```python
from build123d import *

# Parameters (mm, degrees)
SKETCH1_R               = 10
SKETCH1_R_2             = 4
BOSS_EXTRUDE1_DEPTH     = 30
SKETCH2_R               = 2
CUT_EXTRUDE1_DEPTH      = 11
CUT_EXTRUDE1_DEPTH_BACK = 11
FILLET1_R               = 1


with BuildPart() as part:
    # Sketch1 → Boss-Extrude1 (new body)
    with BuildSketch(Plane(origin=(0, 0, 0), x_dir=(1, 0, 0), z_dir=(0, 1, 0))):
        Circle(SKETCH1_R)
        Circle(SKETCH1_R_2, mode=Mode.SUBTRACT)
    extrude(amount=BOSS_EXTRUDE1_DEPTH)

    # Sketch2 → Cut-Extrude1 (cut, two sides)
    with BuildSketch(Plane(origin=(0, 0, 0), x_dir=(0, 0, -1), z_dir=(1, 0, 0))) as cut_extrude1_sk:
        with Locations((6.5, 25.5)):
            Circle(SKETCH2_R)
        with Locations((-6.5, 4.5)):
            Circle(SKETCH2_R)
    extrude(amount=CUT_EXTRUDE1_DEPTH, mode=Mode.SUBTRACT)
    extrude(cut_extrude1_sk.sketch, amount=-CUT_EXTRUDE1_DEPTH_BACK, mode=Mode.SUBTRACT)

    # Fillet1
    fillet1_edges = [part.edges().sort_by_distance(p)[0] for p in [
        (-10, 0, 0),
        (-10, 30, 0),
        (-4, 0, 0),
        (-4, 30, 0),
    ]]
    fillet(fillet1_edges, radius=FILLET1_R)


solid = part.part
```
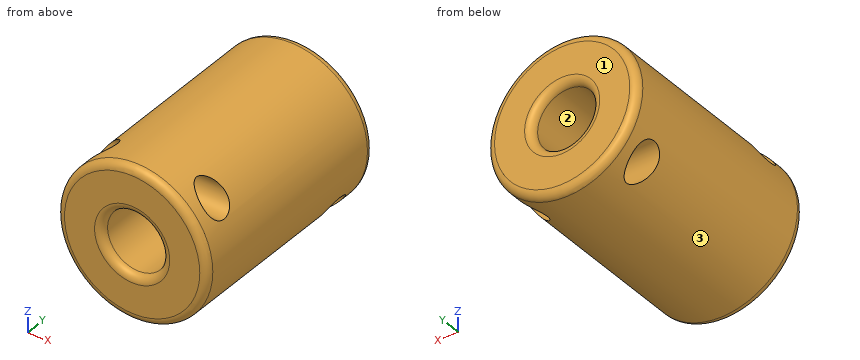
Source: CAD feature listing. Evaluate the final solid. Frame: model axes, mm. Face numbers are marked on the shaded views. Give positions to 0.01 mm unless a question says otherwise; leave off trailing zeros. Write each loop counter-clockwise with the first axis right and the second up, starting at its lowest first coordinate (ties: lowest second). Pieces come first, ordered by that corner, then holes.
1. Section query A-A (z = 0). Return the cut outline in (x, y).
2. Section query C-C (x = -2.25). Count the separate pieces of the cut face and the enclosed holes in it, then the cut area to 3 significant figures.
3. First-contact query: pin 1 (12 mm diameter, centred on x = -7, y = 6.5, fed in from +Z); pin 2 (1.5 mm diameter, centred on x = 4, y = 17, fed in from +Z); pin 3 (5 mm diameter, centred on y = 4.5, z = 6.5, fed in from -X); pin 4 (3.5 mm diameter, centred on y = 25.5, z = -6.5, fed in from -X). Flat tips, straight axial feed; report the tip coordinate or a pass-through.
4. Section query D-D (y = 21). Return the cut outline in (x, z).
5. Pull-direction query (Z, two-part tool) for the marked faces 1, 2 and 3; classes: +Z half, -Z half, draft (parallel to the pull), parting line (faces both ways), or undercut.
6. Material intervals for line 1 along Y through (x, z) = (6.25, 6.5); line 2 along Y through (x, z) = (-3.25, -6.5); line 3 along X through (y, z) = (3, 0), sorted ascending.
7. Section query B-B (y = 3.25). Return the cut outline in (x, z).
Output values:
1. outline: (-10, 1) arc R1 ccw to (-9, 0) - (-5, 0) arc R1 ccw to (-4, 1) - (-4, 29) arc R1 ccw to (-5, 30) - (-9, 30) arc R1 ccw to (-10, 29) - close; (4, 1) arc R1 ccw to (5, 0) - (9, 0) arc R1 ccw to (10, 1) - (10, 29) arc R1 ccw to (9, 30) - (5, 30) arc R1 ccw to (4, 29) - close
2. separate pieces: 2
2. enclosed holes: 2
2. area: 359 mm2
3. pin 1: stops at z = 9.95
3. pin 2: stops at z = 9.46
3. pin 3: stops at x = -9.17
3. pin 4: passes through
4. outline: circle Ø20 at (0, 0); hole circle Ø8 at (0, 0)
5. face 1: draft
5. face 2: undercut
5. face 3: parting line
6. line 1: y = 0 to 2.5, 6.5 to 30
6. line 2: y = 0 to 23.5, 27.5 to 30
6. line 3: x = -10 to -4, 4 to 10
7. outline: (-8.7, 4.94) arc R10 ccw (long way) to (8.7, 4.94) - close; (-5.92, 8.06) - (5.92, 8.06) arc R10 ccw to start; hole circle Ø8 at (0, 0)
